For this review, take the finished solid that the model builds, in its own axes (mm). A direction names the side the tool comes from. Round coordinates to 2 decimals unless told otherwise and drop trailing zeros. Write each loop counter-clockwise with the first axis right and the second up, starting at its lowest first coordinate (ties: lowest second). Pieces come first, ordered by that corner, then holes.
from build123d import *


with BuildPart() as f4:
    # F0 (on Right) → F4 (revolve)
    with BuildSketch(Plane.YZ):
        with BuildLine():
            Line((-52.6758568757, 24.765), (-59.055, 21.082))
            Line((-59.055, 21.082), (-20.955, 21.082))
            Line((-20.955, 21.082), (-20.955, 15.875))
            Line((-20.955, 15.875), (0, 15.875))
            ThreePointArc((0, 15.875), (11.2253201513, 11.2253201513), (15.875, 0))
            Line((15.875, 0), (24.765, 0))
            ThreePointArc((24.765, 0), (17.5114994361, 17.5114994361), (0, 24.765))
            Line((0, 24.765), (-52.6758568757, 24.765))
        make_face()
        with BuildLine():
            Line((-20.955, 21.082), (-59.055, 21.082))
            Line((-59.055, 21.082), (-59.055, 0))
            Line((-59.055, 0), (0, 0))
            Line((0, 0), (10.5189766587, 0))
            Line((10.5189766587, 0), (15.875, 0))
            ThreePointArc((15.875, 0), (11.2253201513, 11.2253201513), (0, 15.875))
            Line((0, 15.875), (-20.955, 15.875))
            Line((-20.955, 15.875), (-20.955, 21.082))
        make_face()
    revolve(axis=Axis((0, -21.59, 0), (0, 1, 0)))

    # F1 (on Right) → F5 (revolve)
    with BuildSketch(Plane.YZ):
        with BuildLine():
            Line((-24.765, -52.6758568757), (-21.082, -59.055))
            Line((-21.082, -59.055), (-21.082, -20.955))
            Line((-21.082, -20.955), (-15.875, -20.955))
            Line((-15.875, -20.955), (-15.875, 0))
            ThreePointArc((-15.875, 0), (-11.2253201513, 11.2253201513), (0, 15.875))
            Line((0, 15.875), (0, 24.765))
            ThreePointArc((0, 24.765), (-17.5114994361, 17.5114994361), (-24.765, 0))
            Line((-24.765, 0), (-24.765, -52.6758568757))
        make_face()
        with BuildLine():
            Line((-21.082, -20.955), (-21.082, -59.055))
            Line((-21.082, -59.055), (0, -59.055))
            Line((0, -59.055), (0, 0))
            Line((0, 0), (0, 15.875))
            ThreePointArc((0, 15.875), (-11.2253201513, 11.2253201513), (-15.875, 0))
            Line((-15.875, 0), (-15.875, -20.955))
            Line((-15.875, -20.955), (-21.082, -20.955))
        make_face()
    revolve(axis=Axis((0, 0, -21.59), (0, 0, 1)))

    # F2 (on Right) → F6 (revolve)
    with BuildSketch(Plane.YZ):
        with BuildLine():
            Line((52.6758568757, -24.765), (59.055, -21.082))
            Line((59.055, -21.082), (20.955, -21.082))
            Line((20.955, -21.082), (20.955, -15.875))
            Line((20.955, -15.875), (0, -15.875))
            ThreePointArc((0, -15.875), (-11.2253201513, -11.2253201513), (-15.875, 0))
            Line((-15.875, 0), (-24.765, 0))
            ThreePointArc((-24.765, 0), (-17.5114994361, -17.5114994361), (0, -24.765))
            Line((0, -24.765), (52.6758568757, -24.765))
        make_face()
        with BuildLine():
            Line((20.955, -21.082), (59.055, -21.082))
            Line((59.055, -21.082), (59.055, 0))
            Line((59.055, 0), (10.5189766587, 0))
            Line((10.5189766587, 0), (0, 0))
            Line((0, 0), (-15.875, 0))
            ThreePointArc((-15.875, 0), (-11.2253201513, -11.2253201513), (0, -15.875))
            Line((0, -15.875), (20.955, -15.875))
            Line((20.955, -15.875), (20.955, -21.082))
        make_face()
    revolve(axis=Axis((0, 21.59, 0), (0, -1, 0)))

    # F3 (on Right) → F7 (revolve)
    with BuildSketch(Plane.YZ):
        with BuildLine():
            Line((24.765, 52.6758568757), (21.082, 59.055))
            Line((21.082, 59.055), (21.082, 20.955))
            Line((21.082, 20.955), (15.875, 20.955))
            Line((15.875, 20.955), (15.875, 0))
            ThreePointArc((15.875, 0), (11.2253201513, -11.2253201513), (0, -15.875))
            Line((0, -15.875), (0, -24.765))
            ThreePointArc((0, -24.765), (17.5114994361, -17.5114994361), (24.765, 0))
            Line((24.765, 0), (24.765, 52.6758568757))
        make_face()
        with BuildLine():
            Line((21.082, 20.955), (21.082, 59.055))
            Line((21.082, 59.055), (0, 59.055))
            Line((0, 59.055), (0, 9.2996467855))
            Line((0, 9.2996467855), (0, 0))
            Line((0, 0), (0, -15.875))
            ThreePointArc((0, -15.875), (11.2253201513, -11.2253201513), (15.875, 0))
            Line((15.875, 0), (15.875, 20.955))
            Line((15.875, 20.955), (21.082, 20.955))
        make_face()
    revolve(axis=Axis((0, 0, 21.59), (0, 0, -1)))

    # F0 (on Right) → F8 (revolve, cut)
    with BuildSketch(Plane.YZ):
        with BuildLine():
            Line((-20.955, 21.082), (-59.055, 21.082))
            Line((-59.055, 21.082), (-59.055, 0))
            Line((-59.055, 0), (0, 0))
            Line((0, 0), (10.5189766587, 0))
            Line((10.5189766587, 0), (15.875, 0))
            ThreePointArc((15.875, 0), (11.2253201513, 11.2253201513), (0, 15.875))
            Line((0, 15.875), (-20.955, 15.875))
            Line((-20.955, 15.875), (-20.955, 21.082))
        make_face()
    revolve(axis=Axis((0, -21.59, 0), (0, 1, 0)), mode=Mode.SUBTRACT)

    # F1 (on Right) → F9 (revolve, cut)
    with BuildSketch(Plane.YZ):
        with BuildLine():
            Line((-21.082, -20.955), (-21.082, -59.055))
            Line((-21.082, -59.055), (0, -59.055))
            Line((0, -59.055), (0, 0))
            Line((0, 0), (0, 15.875))
            ThreePointArc((0, 15.875), (-11.2253201513, 11.2253201513), (-15.875, 0))
            Line((-15.875, 0), (-15.875, -20.955))
            Line((-15.875, -20.955), (-21.082, -20.955))
        make_face()
    revolve(axis=Axis((0, 0, -21.59), (0, 0, 1)), mode=Mode.SUBTRACT)

    # F2 (on Right) → F10 (revolve, cut)
    with BuildSketch(Plane.YZ):
        with BuildLine():
            Line((20.955, -21.082), (59.055, -21.082))
            Line((59.055, -21.082), (59.055, 0))
            Line((59.055, 0), (10.5189766587, 0))
            Line((10.5189766587, 0), (0, 0))
            Line((0, 0), (-15.875, 0))
            ThreePointArc((-15.875, 0), (-11.2253201513, -11.2253201513), (0, -15.875))
            Line((0, -15.875), (20.955, -15.875))
            Line((20.955, -15.875), (20.955, -21.082))
        make_face()
    revolve(axis=Axis((0, 21.59, 0), (0, -1, 0)), mode=Mode.SUBTRACT)

    # F3 (on Right) → F11 (revolve, cut)
    with BuildSketch(Plane.YZ):
        with BuildLine():
            Line((21.082, 20.955), (21.082, 59.055))
            Line((21.082, 59.055), (0, 59.055))
            Line((0, 59.055), (0, 9.2996467855))
            Line((0, 9.2996467855), (0, 0))
            Line((0, 0), (0, -15.875))
            ThreePointArc((0, -15.875), (11.2253201513, -11.2253201513), (15.875, 0))
            Line((15.875, 0), (15.875, 20.955))
            Line((15.875, 20.955), (21.082, 20.955))
        make_face()
    revolve(axis=Axis((0, 0, 21.59), (0, 0, -1)), mode=Mode.SUBTRACT)


solid = f4.part
(1) For line 1 along Y through (x, z) = (0, 39) (3 decimals); line 2 along X through (y, z) = (-1, -43.5), list the stretches that pass through material, from the lowest coordinate up.
Geometry check:
line 1: y = -24.765 to -21.082, 21.082 to 24.765
line 2: x = -24.74 to -21.06, 21.06 to 24.74
(2) We need section B-B, the plane y = 40. Give the boundary of the cut face in (x, z) (3 decimals).
Geometry check:
outline: circle Ø49.53 at (0, 0); hole circle Ø42.164 at (0, 0)
(3) We need section A-A, the plane x = 0. State how many separate pieces and enclosed holes the cut face has, and give its area (3 significant figures).
Geometry check:
separate pieces: 8
enclosed holes: 0
area: 1,070 mm2
(4) Mouldability with a two-part tool opening along X and no side actions: class faces 1 (the face through (6.33, -20.11, -40.27)), 2 (the face through (16.74, 18.25, -32.56)) as pulls with the +X half, pulls with the -X half, needs draft (parallel to the pull), parting line crosses it, or undercut.
Geometry check:
face 1: undercut
face 2: parting line crosses it
(5) For faces 3 (the face through (6.33, 20.11, 40.27)), 4 (the face through (-9, 14, -20.955)), 5 (the face through (-1.09, -31.82, -24.74)), 6 (the face through (16.74, 32.56, 18.25)), list the 3-axis set-ups (+Z, -Z, +X, -X, +Y, -Y) from which the entire face can be reached by the end or side of a thin tool; tool diameter is ignored.
Geometry check:
face 3: +Z
face 4: -Z
face 5: -Y
face 6: +Y
(6) For pin 1 Ø3 at (x, z) = (-11, -16.5) entering from -Y (3 decimals); pin 2 Ø12 at (x, y) = (-1, -45) entering from -Z (3 decimals); pin 3 Ø21 at (x, z) = (3.5, -3.5) entering from -Y; pin 4 Ø4 at (y, z) = (15, 28.5) entering from -X, all flat-tipped, find the tip position at first contact; note any pin that passes through.
Geometry check:
pin 1: stops at y = -59.055
pin 2: stops at z = -24.765
pin 3: passes through
pin 4: stops at x = -21.08
